from build123d import *

# Parameters (mm, degrees)
BOSS_EXTRUDE1_DEPTH             = 18.796
CUT_EXTRUDE1_DEPTH              = 16.256
FILLET1_R                       = 2.54
CUT_EXTRUDE2_DEPTH              = 57.332624837
CUT_EXTRUDE2_DEPTH_BACK         = 57.332624837
SKETCH3_W                       = 32.258
SKETCH3_H                       = 8.128
SKETCH5_W                       = 26.924
SKETCH5_H                       = 34.29
CUT_EXTRUDE4_DEPTH              = 1.524
SKETCH6_W                       = 16.764
SKETCH6_H                       = 24.13
CUT_EXTRUDE5_DEPTH              = 1.524
SKETCH8_W                       = 12.7
SKETCH8_H                       = 0.508
BOSS_EXTRUDE3_DEPTH             = 4.064
SKETCH9_W                       = 12.7
SKETCH9_H                       = 1.016
BOSS_EXTRUDE4_DEPTH             = 0.762
FILLET2_R                       = 0.762
SKETCH10_W                      = 12.7
SKETCH10_H                      = 1.016
BOSS_EXTRUDE5_DEPTH             = 0.762
FILLET3_R                       = 0.762
SKETCH11_W                      = 1.778
SKETCH11_H                      = 4.064
BOSS_EXTRUDE6_DEPTH             = 3.556
BOSS_EXTRUDE6_DIRECTION_2_REACH = 58.333
FILLET4_RADIUS                  = 2.032
FILLET4_LENGTH                  = 1.778
SKETCH12_R                      = 1.143
CUT_EXTRUDE7_DEPTH              = 4.064
CUT_EXTRUDE8_DEPTH              = 0.762
SKETCH13_W                      = 2.54
SKETCH13_H                      = 5.08
BOSS_EXTRUDE7_DEPTH             = 16.256
SKETCH15_W                      = 11.176
SKETCH15_H                      = 2.54
BOSS_EXTRUDE8_DEPTH             = 3.556


with BuildPart() as part:
    # Sketch1 → Boss-Extrude1 (new body)
    with BuildSketch(Plane.XY):
        with BuildLine():
            Line((-21.209, -23.749), (21.209, -23.749))
            ThreePointArc((21.209, -23.749), (23.005051224, -23.005051224), (23.749, -21.209))
            Line((23.749, -21.209), (23.749, 21.209))
            ThreePointArc((23.749, 21.209), (23.005051224, 23.005051224), (21.209, 23.749))
            Line((21.209, 23.749), (-21.209, 23.749))
            ThreePointArc((-21.209, 23.749), (-23.005051224, 23.005051224), (-23.749, 21.209))
            Line((-23.749, 21.209), (-23.749, -21.209))
            ThreePointArc((-23.749, -21.209), (-23.005051224, -23.005051224), (-21.209, -23.749))
        make_face()
    extrude(amount=BOSS_EXTRUDE1_DEPTH)

    # Sketch2 → Cut-Extrude1 (cut)
    with BuildSketch(Plane.XY.offset(18.796)):
        with BuildLine():
            Line((19.939, -22.479), (-19.939, -22.479))
            ThreePointArc((-19.939, -22.479), (-21.735051224, -21.735051224), (-22.479, -19.939))
            Line((-22.479, -19.939), (-22.479, 19.939))
            ThreePointArc((-22.479, 19.939), (-21.735051224, 21.735051224), (-19.939, 22.479))
            Line((-19.939, 22.479), (19.939, 22.479))
            ThreePointArc((19.939, 22.479), (21.735051224, 21.735051224), (22.479, 19.939))
            Line((22.479, 19.939), (22.479, -19.939))
            ThreePointArc((22.479, -19.939), (21.735051224, -21.735051224), (19.939, -22.479))
        make_face()
    extrude(amount=-CUT_EXTRUDE1_DEPTH, mode=Mode.SUBTRACT)

    # Fillet1
    fillet1_edges = [part.edges().sort_by_distance(p)[0] for p in [
        (0, -23.749, 0),
        (-23.005051224, -23.005051224, 0),
        (-23.749, 0, 0),
        (-23.005051224, 23.005051224, 0),
        (0, 23.749, 0),
        (23.005051224, 23.005051224, 0),
        (23.749, 0, 0),
        (23.005051224, -23.005051224, 0),
    ]]
    fillet(fillet1_edges, radius=FILLET1_R)

    # Sketch3 → Cut-Extrude2 (cut, two sides: drawn at the far end of the back side and taken through both)
    with BuildSketch(Plane(origin=(0, 23.749, 0), x_dir=(1, 0, 0), z_dir=(0, 1, 0)).offset(-CUT_EXTRUDE2_DEPTH_BACK)):
        with Locations((0, -18.796)):
            Rectangle(SKETCH3_W, SKETCH3_H)
    extrude(amount=CUT_EXTRUDE2_DEPTH + CUT_EXTRUDE2_DEPTH_BACK, mode=Mode.SUBTRACT)

    # Sketch5 → Cut-Extrude4 (cut)
    with BuildSketch(Plane(origin=(0, 0, 0), x_dir=(-1, 0, 0), z_dir=(0, 0, -1))):
        with Locations((-1.143, 0)):
            Rectangle(SKETCH5_W, SKETCH5_H)
    extrude(amount=-CUT_EXTRUDE4_DEPTH, mode=Mode.SUBTRACT)

    # Sketch6 → Cut-Extrude5 (cut)
    with BuildSketch(Plane(origin=(0, 0, 1.524), x_dir=(-1, 0, 0), z_dir=(0, 0, -1))):
        with Locations((-1.143, 0)):
            Rectangle(SKETCH6_W, SKETCH6_H)
    extrude(amount=-CUT_EXTRUDE5_DEPTH, mode=Mode.SUBTRACT)

    # Sketch8 → Boss-Extrude3 (add)
    with BuildSketch(Plane.XY.offset(14.732)):
        with Locations((0, 22.733)):
            Rectangle(SKETCH8_W, SKETCH8_H)
        with Locations((0, -22.733)):
            Rectangle(SKETCH8_W, SKETCH8_H)
    extrude(amount=BOSS_EXTRUDE3_DEPTH)

    # Sketch9 → Boss-Extrude4 (add)
    with BuildSketch(Plane(origin=(0, 22.987, 0), x_dir=(1, 0, 0), z_dir=(0, 1, 0))):
        with Locations((0, -18.288)):
            Rectangle(SKETCH9_W, SKETCH9_H)
    extrude(amount=BOSS_EXTRUDE4_DEPTH)

    # Fillet2
    fillet2_edges = [part.edges().sort_by_distance(p)[0] for p in [
        (0, 22.987, 17.78),
    ]]
    fillet(fillet2_edges, radius=FILLET2_R - 0.0001)  # a hair under: the kernel refuses the full size

    # Sketch10 → Boss-Extrude5 (add)
    with BuildSketch(Plane.XZ.offset(22.987)):
        with Locations((0, 18.288)):
            Rectangle(SKETCH10_W, SKETCH10_H)
    extrude(amount=BOSS_EXTRUDE5_DEPTH)

    # Fillet3
    fillet3_edges = [part.edges().sort_by_distance(p)[0] for p in [
        (0, -22.987, 17.78),
    ]]
    fillet(fillet3_edges, radius=FILLET3_R - 0.0001)  # a hair under: the kernel refuses the full size

    # Sketch11 → Boss-Extrude6 (add)
    with BuildSketch(Plane.ZY.offset(23.749)):
        with Locations((17.907, -21.717)):
            Rectangle(SKETCH11_W, SKETCH11_H)
    extrude(amount=BOSS_EXTRUDE6_DEPTH)

    # Sketch11 → Boss-Extrude6 direction 2 (add, up to next)
    with BuildSketch(Plane.ZY.offset(23.749), mode=Mode.PRIVATE) as boss_extrude6_direction_2_sk1:
        with Locations((17.907, -21.717)):
            Rectangle(SKETCH11_W, SKETCH11_H)
    boss_extrude6_direction_2_tool1 = extrude(boss_extrude6_direction_2_sk1.sketch, amount=-BOSS_EXTRUDE6_DIRECTION_2_REACH, mode=Mode.PRIVATE) - part.part
    add(boss_extrude6_direction_2_tool1.solids().sort_by_distance((-23.749, -21.717, 17.907))[0])

    # Fillet4: full round fillet: the end face becomes a half cylinder, R = half its width
    fillet4_face = Plane((-27.305, -21.717, 17.907), x_dir=(0, 0, -1), z_dir=(-1, 0, 0))  # on the end face: x along it, z out of the body
    fillet4_slab = fillet4_face.offset(-FILLET4_RADIUS / 2) * Box(FILLET4_LENGTH, 2 * FILLET4_RADIUS, FILLET4_RADIUS, mode=Mode.PRIVATE)  # the body's end, R deep
    fillet4_round = Plane((-25.273, -21.717, 17.907), x_dir=(-1, 0, 0), z_dir=(0, 0, -1)) * Cylinder(FILLET4_RADIUS, FILLET4_LENGTH, mode=Mode.PRIVATE)  # its axis R under the face
    add(fillet4_slab - fillet4_round, mode=Mode.SUBTRACT)

    # Sketch12 → Cut-Extrude7 (cut)
    with BuildSketch(Plane(origin=(0, 0, 17.018), x_dir=(-1, 0, 0), z_dir=(0, 0, -1))):
        with Locations((25.273, -21.717)):
            Circle(SKETCH12_R)
    extrude(amount=-CUT_EXTRUDE7_DEPTH, mode=Mode.SUBTRACT)

    # Sketch7 → Cut-Extrude8 (cut)
    with BuildSketch(Plane(origin=(0, 0, 0), x_dir=(-1, 0, 0), z_dir=(0, 0, -1))):
        with BuildLine():
            Line((19.939, 17.145), (21.209, 17.145))
            ThreePointArc((21.209, 17.145), (17.399, 20.955), (13.589, 17.145))
            Line((13.589, 17.145), (14.859, 17.145))
            ThreePointArc((14.859, 17.145), (17.399, 19.685), (19.939, 17.145))
        make_face()
        with BuildLine():
            Line((21.209, 15.875), (16.129, 15.875))
            ThreePointArc((16.129, 15.875), (13.589, 13.335), (16.129, 10.795))
            Line((16.129, 10.795), (21.209, 10.795))
            Line((21.209, 10.795), (21.209, 12.065))
            Line((21.209, 12.065), (16.129, 12.065))
            ThreePointArc((16.129, 12.065), (14.859, 13.335), (16.129, 14.605))
            Line((16.129, 14.605), (21.209, 14.605))
            Line((21.209, 14.605), (21.209, 15.875))
        make_face()
        Polygon((13.589, 9.525), (21.209, 9.525), (21.209, 5.715), (19.939, 5.715), (19.939, 8.255), (18.034, 8.255), (18.034, 6.985), (16.764, 6.985), (16.764, 8.255), (13.589, 8.255), align=None)
        Polygon((13.589, 4.445), (21.209, 4.445), (21.209, 0.635), (19.939, 0.635), (19.939, 3.175), (18.034, 3.175), (18.034, 1.905), (16.764, 1.905), (16.764, 3.175), (13.589, 3.175), align=None)
        Polygon((21.209, -0.635), (13.589, -0.635), (13.589, -4.445), (14.859, -4.445), (14.859, -1.905), (21.209, -1.905), align=None)
        Polygon((13.589, -5.715), (21.209, -5.715), (21.209, -9.525), (19.939, -9.525), (19.939, -6.985), (18.034, -6.985), (18.034, -8.255), (16.764, -8.255), (16.764, -6.985), (14.859, -6.985), (14.859, -9.525), (13.589, -9.525), align=None)
        with BuildLine():
            Line((18.9865, -13.97), (18.9865, -15.24))
            ThreePointArc((18.9865, -15.24), (20.558044821, -11.445955179), (16.764, -13.0175))
            ThreePointArc((16.764, -13.0175), (15.137980791, -13.691019209), (15.8115, -12.065))
            Line((15.8115, -12.065), (15.8115, -10.795))
            ThreePointArc((15.8115, -10.795), (14.239955179, -14.589044821), (18.034, -13.0175))
            ThreePointArc((18.034, -13.0175), (19.660019209, -12.343980791), (18.9865, -13.97))
        make_face()
        with BuildLine():
            Line((15.8115, -17.78), (15.8115, -16.51))
            ThreePointArc((15.8115, -16.51), (14.239955179, -20.304044821), (18.034, -18.7325))
            ThreePointArc((18.034, -18.7325), (19.660019209, -18.058980791), (18.9865, -19.685))
            Line((18.9865, -19.685), (18.9865, -20.955))
            ThreePointArc((18.9865, -20.955), (20.558044821, -17.160955179), (16.764, -18.7325))
            ThreePointArc((16.764, -18.7325), (15.137980791, -19.406019209), (15.8115, -17.78))
        make_face()
    extrude(amount=-CUT_EXTRUDE8_DEPTH, mode=Mode.SUBTRACT)

    # Sketch13 → Boss-Extrude7 (add)
    with BuildSketch(Plane.XY.offset(2.54)):
        with Locations((17.907, -14.859)):
            Rectangle(SKETCH13_W, SKETCH13_H)
    extrude(amount=BOSS_EXTRUDE7_DEPTH)

    # Sketch15 → Boss-Extrude8 (add)
    with BuildSketch(Plane(origin=(19.177, 0, 0), x_dir=(0, 0, -1), z_dir=(1, 0, 0))):
        with Locations((-8.128, -14.859)):
            Rectangle(SKETCH15_W, SKETCH15_H)
    extrude(amount=BOSS_EXTRUDE8_DEPTH)


solid = part.part
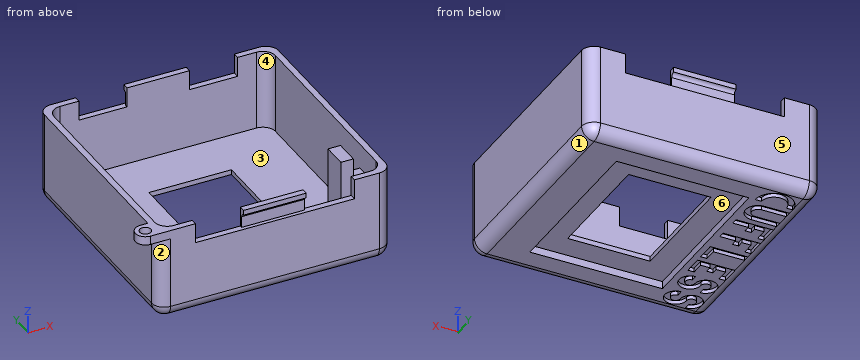
Input: part model. Units: mm. Frame: model coordinates. Face numbers are marked on the shaded views. A direction names the side the tool comes from. Round coordinates to 2 decimals unless told otherwise and drop trailing zeros. Write each loop counter-clockwise with the first axis right and the second up, starting at its lowest first coordinate (ties: lowest second). Pieces come first, ordered by that corner, then holes.
1) Cut plane C-C (x = 18.5). Return the cut outline in (y, z), then the cut area to 3 significant figures.
2) Draft query along X for the marked faces 1, 2 and 3. Return one class per face: pulls with the +X half, pulls with the -X half, needs draft (parallel to the pull), parting line crosses it, or undercut.
3) Reachability of the marked faces 4, 5 and 6 from +Z, -Z, +X, -X, +Y, -Y: full face, straight path, thin tool, end or side. Return the list, or none.
4) Contact query for flat-ended pins moving along their axis: P1, Ø6, axis at y = 14.5, z = 16, coming from the -X side; P2, Ø0.8, axis at y = -8, z = 0.5, coming from the +X side; P3, Ø0.6, axis at x = -17.5, z = 0.5, coming from the -Y side. Output: stop coordinate, or through.
5) Ray query, L1, parallel to X at y = -13, z = 15; L2, parallel to X at y = -1, z = 2.5 (3 decimals); L3, parallel to X at y = 17.5, z = 16.5. Return the intervals inside material, ascending.
6) Cut plane B-B (z = 11). Return the cut outline in (x, y).
7) Cut plane D-D (x = -8). Return the cut outline in (y, z) (3 decimals).
8) Cut plane A-A (y = -3.5). Return the cut outline in (x, z) (3 decimals), then the cut area to 3 significant figures.
Geometry says:
1. outline: (-23.75, 2.54) arc R2.54 ccw to (-21.21, 0) - (21.21, 0) arc R2.54 ccw to (23.75, 2.54) - (23.75, 18.8) - (22.48, 18.8) - (22.48, 2.54) - (-12.32, 2.54) - (-12.32, 18.8) - (-17.4, 18.8) - (-17.4, 2.54) - (-22.48, 2.54) - (-22.48, 18.8) - (-23.75, 18.8) - close
1. area: 242 mm2
2. face 1: pulls with the +X half
2. face 2: pulls with the -X half
2. face 3: undercut
3. face 4: +Z
3. face 5: +Z, -Z, +X, -X, +Y
3. face 6: -Z
4. P1: stops at x = -23.75
4. P2: stops at x = 23.15
4. P3: stops at y = -23.06
5. L1: x = -23.75 to -22.48, 16.64 to 19.18, 22.48 to 23.75
5. L2: x = -23.749 to -7.239, 9.525 to 23.749
5. L3: x = -23.75 to -22.48, 22.48 to 23.75
6. outline: (-23.75, -21.21) arc R2.54 ccw to (-21.21, -23.75) - (21.21, -23.75) arc R2.54 ccw to (23.75, -21.21) - (23.75, 21.21) arc R2.54 ccw to (21.21, 23.75) - (-21.21, 23.75) arc R2.54 ccw to (-23.75, 21.21) - close; hole (-22.48, -19.94) arc R2.54 ccw to (-19.94, -22.48) - (19.94, -22.48) arc R2.54 ccw to (22.48, -19.94) - (22.48, -16.13) - (19.18, -16.13) - (19.18, -17.4) - (16.64, -17.4) - (16.64, -12.32) - (19.18, -12.32) - (19.18, -13.59) - (22.48, -13.59) - (22.48, 19.94) arc R2.54 ccw to (19.94, 22.48) - (-19.94, 22.48) arc R2.54 ccw to (-22.48, 19.94) - close
7. outline: (-23.749, 2.54) arc R2.54 ccw to (-21.209, 0) - (-17.145, 0) - (-17.145, 1.524) - (17.145, 1.524) - (17.145, 0) - (21.209, 0) arc R2.54 ccw to (23.749, 2.54) - (23.749, 14.732) - (22.479, 14.732) - (22.479, 2.54) - (-22.479, 2.54) - (-22.479, 14.732) - (-23.749, 14.732) - close
8. outline: (-23.749, 2.54) arc R2.54 ccw to (-21.209, 0) - (-14.859, 0) - (-14.859, 0.762) - (-13.589, 0.762) - (-13.589, 0) - (-12.319, 0) - (-12.319, 1.524) - (-7.239, 1.524) - (-7.239, 2.54) - (-22.479, 2.54) - (-22.479, 18.796) - (-23.749, 18.796) - close; (9.525, 1.524) - (14.605, 1.524) - (14.605, 0) - (21.209, 0) arc R2.54 ccw to (23.749, 2.54) - (23.749, 18.796) - (22.479, 18.796) - (22.479, 2.54) - (9.525, 2.54) - close
8. area: 100 mm2
